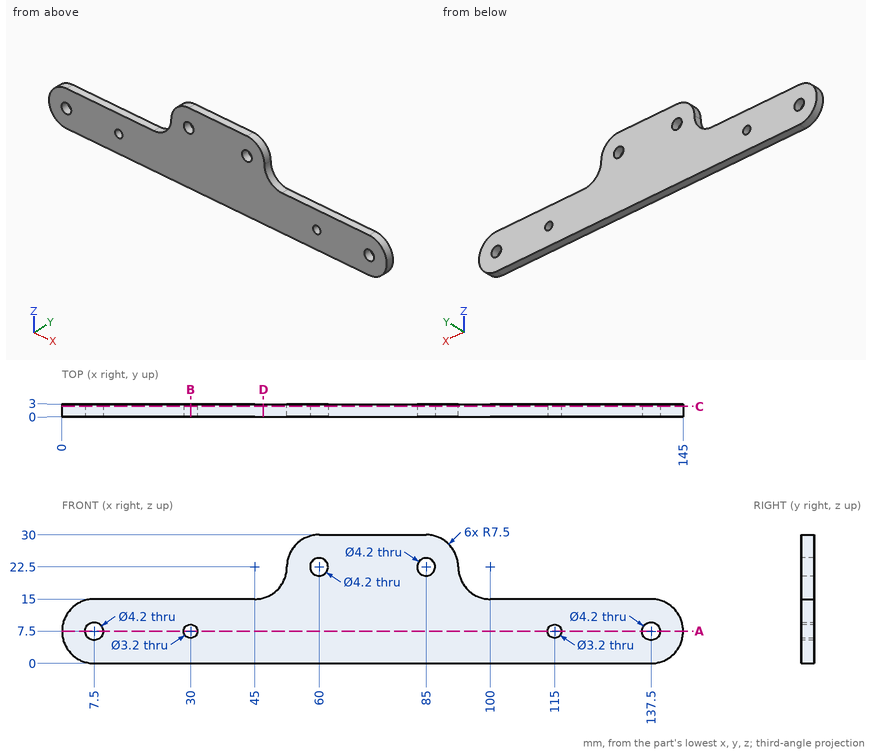
Could you check a few things on this drawing? It's one solid part, dimensions in mm from its lowest x, y, z. Give positions to 0.01 mm unless a question says otherwise; leave off trailing zeros. Order: outer loops, then holes, each group sorted by start corner. A loop starts at its lowest first (then second) coordinate and runs counter-clockwise, first axis right, second up. Notation, with made-up numbers: (20.25, -14) - (60.25, -14) arc R22 cw to (60.25, -2) - close; hole circle Ø5 at (58, -26). An arc over 180 degrees is marked (long way). Return JSON: item names as keys, results as strings. Group by question number.
Q1. Please list where these lines run through material, in increasing order: line 1 along X through (y, z) = (1.8, 7.5); line 2 along Z through (x, y) = (115, 0.75); line 3 along X through (y, z) = (1.4, 7). Write a range as [from, to].
Q2. Suppose I cut it at C-C, the plane y = 2.45. Please give me the cut outline in (x, z).
Q3. Will these pins go through, and if not, where does the flat tip stop? pin 1 Ø1.5 at (x, y) = (31, 1.5) entering from +Z; pin 2 Ø3 at (x, z) = (115, 7.5) entering from -Y.
Q4. Suppose I cut it at D-D, the plane x = 47. Please give me the cut outline in (y, z), and give its area (3 significant figures).
Q5. Suppose I cut it at B-B, the plane x = 30. Please give me the cut outline in (y, z).
Q6. Suppose I cut it at A-A, the plane z = 7.5. Please give me the cut outline in (x, y).
Resolved:
{
 "1": {"line 1": "x = [0, 5.4], [9.6, 28.4], [31.6, 113.4], [116.6, 135.4], [139.6, 145]", "line 2": "z = [0, 5.9], [9.1, 15]", "line 3": "x = [0.02, 5.46], [9.54, 28.48], [31.52, 113.48], [116.52, 135.46], [139.54, 144.98]"},
 "2": {"outline": "(7.5, 0) - (137.5, 0) arc R7.5 ccw to (137.5, 15) - (100, 15) arc R7.5 cw to (92.5, 22.5) arc R7.5 ccw to (85, 30) - (60, 30) arc R7.5 ccw to (52.5, 22.5) arc R7.5 cw to (45, 15) - (7.5, 15) arc R7.5 ccw to start; hole circle Ø4.2 at (7.5, 7.5); hole circle Ø3.2 at (30, 7.5); hole circle Ø4.2 at (60, 22.5); hole circle Ø4.2 at (85, 22.5); hole circle Ø3.2 at (115, 7.5); hole circle Ø4.2 at (137.5, 7.5)"},
 "3": {"pin 1": "stops at z = 15", "pin 2": "passes through"},
 "4": {"outline": "(0, 0) - (3, 0) - (3, 15.27) - (0, 15.27) - close", "area": "45.8 mm2"},
 "5": {"outline": "(0, 0) - (3, 0) - (3, 5.9) - (0, 5.9) - close; (0, 9.1) - (3, 9.1) - (3, 15) - (0, 15) - close"},
 "6": {"outline": "(0, 0) - (5.4, 0) - (5.4, 3) - (0, 3) - close; (9.6, 0) - (28.4, 0) - (28.4, 3) - (9.6, 3) - close; (31.6, 0) - (113.4, 0) - (113.4, 3) - (31.6, 3) - close; (116.6, 0) - (135.4, 0) - (135.4, 3) - (116.6, 3) - close; (139.6, 0) - (145, 0) - (145, 3) - (139.6, 3) - close"}
}
